Build history of the part. All positions in model axes, mm. Give positions to 0.01 mm unless a question says otherwise; leave off trailing zeros. Order: outer loops, then holes, each group sorted by start corner. A loop starts at its lowest first (then second) coordinate and runs counter-clockwise, first axis right, second up. Notation, with made-up numbers: (62.25, 51.5) - (105.25, 51.5) arc R12 cw to (105.25, 69.5) - close; hole circle Ø1 at (-19.75, -24). An arc over 180 degrees is marked (long way). Write each question's results on one line, items separated by ' | '. Start each with the question number.
1) Cut at D-D on x = 10.5. List the corners of the cut face in (y, z).
2) Two-plate mould, pull along Z, no slides. Class faces 1 (the face through (2.166, -16.495, 0.269)), 2 (the face through (0, 22, -7)): +Z half, -Z half, draft (parallel to the pull), parting line (faces both ways), or undercut.
3) Cut at C-C on z = 15.5. List the corners of the cut face in (x, y), plus the area to 3 significant figures.
4) Drop flat-ended pins along their axis: pin 1 Ø3 at (y, z) = (21, 2) entering from +X; pin 2 Ø5 at (x, z) = (1.5, -0.5) entering from +Y; pin 3 Ø1.5 at (x, y) = (-2.5, 23) entering from +Z. Give the stop position or say it passes through.
5) Drill centre lines: line 1 along Y through (x, z) = (-1.5, 3); line 2 along Y through (x, z) = (-2, 17.5); line 3 along X through (y, z) = (1.5, -5). Where is each one in solid material? Low to high. Write a range as from..to.
6) Cut at A-A on x = 0. List the corners of the cut face in (y, z), plus the area to 3 significant figures.
7) Cut at B-B on y = 0. List the corners of the cut face in (x, z), plus the area to 3 significant figures.
from build123d import *

# Parameters (mm, degrees)
SKETCH5_R          = 16.637
CUT_EXTRUDE2_DEPTH = 58.401742134
SKETCH6_W          = 10
SKETCH6_H          = 14
CUT_EXTRUDE3_DEPTH = 6


with BuildPart() as part:
    # Sketch4 → Revolve4 (revolve)
    with BuildSketch(Plane(origin=(0, 0, 0), x_dir=(1, 0, 0), z_dir=(0, 1, 0))):
        with BuildLine():
            Line((-12, 22.386603137), (0, 22.386603137))
            Line((0, 22.386603137), (0, -22.386603137))
            Line((0, -22.386603137), (-12, -22.386603137))
            ThreePointArc((-12, -22.386603137), (-25.4, 0), (-12, 22.386603137))
        make_face()
    revolve(axis=Axis((0, 0, -17.487077089), (0, 0, 1)))

    # Sketch5 → Cut-Extrude2 (cut, through all)
    with BuildSketch(Plane.XY.offset(22.386603137)):
        with Locations(Location((0, 0, 0), (0, 0, 180))):
            Circle(SKETCH5_R)
    extrude(amount=-CUT_EXTRUDE2_DEPTH, mode=Mode.SUBTRACT)

    # Sketch6 → Cut-Extrude3 (cut)
    with BuildSketch(Plane(origin=(0, 25.4, 0), x_dir=(1, 0, 0), z_dir=(0, 1, 0))):
        Rectangle(SKETCH6_W, SKETCH6_H)
    extrude(amount=-CUT_EXTRUDE3_DEPTH, mode=Mode.SUBTRACT)


solid = part.part
Results:
1) outline: (-12.91, -19.19) - (-12.91, 19.19) arc R23.13 ccw to start; (12.91, -19.19) arc R23.13 ccw to (12.91, 19.19) - close
2) face 1: draft | face 2: undercut
3) outline: circle Ø40.24 at (0, 0); hole circle Ø33.27 at (0, 0) | area: 403 mm^2
4) pin 1: x = 16.16 | pin 2: y = 19.4 | pin 3: z = 12
5) line 1: -25.18..-16.57, 16.57..19.4 | line 2: -18.3..-16.52, 16.52..18.3 | line 3: -24.86..-16.57, 16.57..24.86
6) outline: (-16.64, -19.19) - (-16.64, 19.19) arc R25.4 ccw to start; (16.64, -19.19) arc R25.4 ccw to (24.42, -7) - (19.4, -7) - (19.4, 7) - (24.42, 7) arc R25.4 ccw to (16.64, 19.19) - close | area: 387 mm^2
7) outline: (-16.64, -19.19) - (-16.64, 19.19) arc R25.4 ccw to start; (16.64, -19.19) arc R25.4 ccw to (16.64, 19.19) - close | area: 467 mm^2
